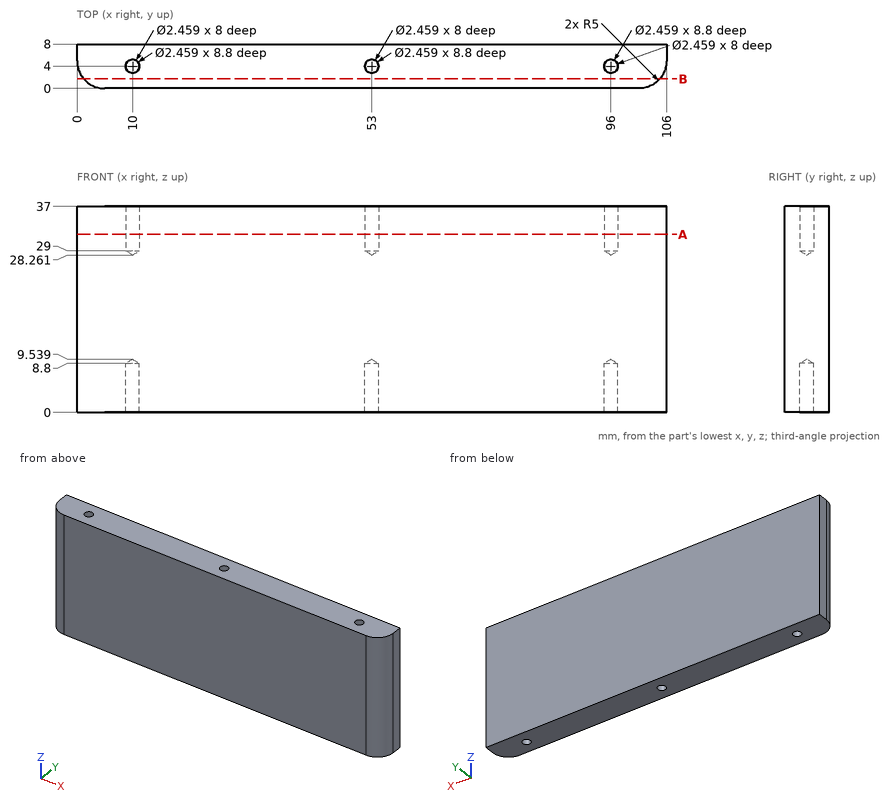
Source: three-view drawing plus pictorial views. Frame: mm from the lowest corner of the part. Give positions to 0.01 mm unless a question says otherwise; leave off trailing zeros. Write each loop counter-clockwise with the first axis right and the second up, starting at its lowest first coordinate (ties: lowest second). Pieces come first, ordered by that corner, then holes.
(1) Cut plane B-B, the plane y = 1.75. Return loops of the section in (x, z).
(2) First-contact query: P1, Ø1.5, axis at x = 10, y = 4, coming from the -Z side; P2, Ø2, axis at x = 96, y = 4, coming from the -Z side; P3, Ø2, axis at y = 2.5, z = 17, coming from the -X side. Flat tips, straight axial feed; report the tip coordinate or a pass-through.
(3) Cut plane A-A, the plane z = 32. Return loops of the section in (x, y).
(4) Ray query, line 1 (Y direction, x = 53, z = 2.5); line 2 (X direction, y = 4, z = 32.5); line 3 (X direction, y = 3.75, z = 30.5). Return the intervals inside material, ascending.
Values follow:
1. outline: (1.2, 0) - (104.8, 0) - (104.8, 37) - (1.2, 37) - close
2. P1: stops at z = 9.09
2. P2: stops at z = 8.94
2. P3: stops at x = 0.23
3. outline: (0, 5) arc R5 ccw to (5, 0) - (101, 0) arc R5 ccw to (106, 5) - (106, 8) - (0, 8) - close; hole circle Ø2.46 at (10, 4); hole circle Ø2.46 at (53, 4); hole circle Ø2.46 at (96, 4)
4. line 1: y = 0 to 2.77, 5.23 to 8
4. line 2: x = 0.1 to 8.77, 11.23 to 51.77, 54.23 to 94.77, 97.23 to 105.9
4. line 3: x = 0.16 to 8.8, 11.2 to 51.8, 54.2 to 94.8, 97.2 to 105.84
